```python
from build123d import *

# Parameters (mm, degrees)
F0_R     = 1.5
F1_DEPTH = 18
F2_R     = 1.5
F3_DEPTH = 6
F4_W     = 3
F4_H     = 1.154314
F5_DEPTH = 4
F6_W     = 2.042234
F6_H     = 1.5
F7_DEPTH = 25


with BuildPart() as f1:
    # F0 (on Top) → F1 (new body)
    with BuildSketch(Plane.XY):
        Circle(F0_R)
    extrude(amount=F1_DEPTH)

    # F2 (on Front) → F3 (join)
    with BuildSketch(Plane.XZ):
        with Locations((0, 4.705742)):
            Circle(F2_R)
    extrude(amount=F3_DEPTH)

    # F4 (on Front) → F5 (join)
    with BuildSketch(Plane.XZ):
        with Locations((0, 6.738564)):
            Rectangle(F4_W, F4_H)
    extrude(amount=-F5_DEPTH)

    # F6 (on face) → F7 (cut)
    with BuildSketch(Plane.XY.offset(7.315721)):
        with Locations((0, 2.75)):
            Rectangle(F6_W, F6_H)
    extrude(amount=-F7_DEPTH, mode=Mode.SUBTRACT)


solid = f1.part
```
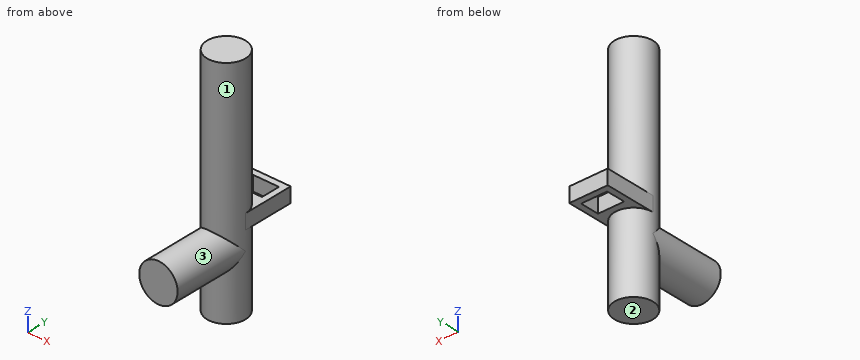
The listing builds one solid part. Answer for the finished solid, in the listing's coordinates (mm). Face numbers are marked on the shaded views. A direction names the side the tool comes from. Coordinates: 2 decimals unless noted, no trailing zeros. Loops run counter-clockwise (first coordinate to the right, second up) from the corner with the lowest first, then second, coordinate; pieces in that order, holes last. Notation, with made-up numbers: M -23.75,5 L 28.25,5 A18 ccw 28.25,28 Z; hole C -5,50 d5. An arc over 180 degrees is marked long. Answer as CSV lines item,"result". Start each with the question number.
(1) The part is cut by section A-A (x = 0). Give the vertices of the cut face in (y, z).
(2) The part is cut by section B-B (y = 2.5). Give the vertices of the cut face in (x, z).
(3) For the marked faces 1, 2 and 3, determine the directions among +Z, -Z, +X, -X, +Y, -Y from which every point of the face is accessible in a straight line to the end or side of a thin tool.
(4) Find the intervals of material crossed by L1, parallel to Y at x = 1.1, z = 11.5; L2, parallel to Z at x = 0.85, y = 1.5; L3, parallel to Y at x = 0.1, z = 9.25, in increasing order. Write a range as [from, to].
(5) Given pin 1 (1 mm diameter, centred on x = 0.5, z = 13.5, fed in from -Y); pin 2 (0.9 mm diameter, centred on x = 0, z = 6.5, fed in from -Y), each flat-ended and moving along its own axis, determine where each tip first touches the part or whether it passes through.
(6) The part is cut by section C-C (z = 13.25). Give the vertices of the cut face in (x, y), and give its area (3 significant figures).
(7) The part is cut by section D-D (x = 1.2). Give the vertices of the cut face in (y, z).
Determined:
1,outline,"M -6,3.21 L -1.5,3.21 L -1.5,0 L 1.5,0 L 1.5,6.16 L 2,6.16 L 2,7.32 L 1.5,7.32 L 1.5,18 L -1.5,18 L -1.5,6.21 L -6,6.21 Z; M 3.5,6.16 L 4,6.16 L 4,7.32 L 3.5,7.32 Z"
2,outline,"M -1.5,6.16 L -1.02,6.16 L -1.02,7.32 L -1.5,7.32 Z; M 1.02,6.16 L 1.5,6.16 L 1.5,7.32 L 1.02,7.32 Z"
3,face 1,"none"
3,face 2,"-Z, +X, -X, +Y, -Y"
3,face 3,"-Y"
4,L1,"[-1.02, 1.02]"
4,L2,"[6.16, 7.32]"
4,L3,"[-1.5, 1.5]"
5,pin 1,"y = -1.5"
5,pin 2,"y = -6"
6,outline,"C 0,0 d3"
6,area,"7.07 mm2"
7,outline,"M -6,3.81 L -0.9,3.81 L -0.9,0 L 0.9,0 L 0.9,6.16 L 4,6.16 L 4,7.32 L 0.9,7.32 L 0.9,18 L -0.9,18 L -0.9,5.61 L -6,5.61 Z"
